Here's how the part is built. I have some questions about the finished solid (model axes, mm). A direction names the side the tool comes from. Coordinates: 2 decimals unless noted, no trailing zeros. Order: outer loops, then holes, each group sorted by start corner. A loop starts at its lowest first (then second) coordinate and runs counter-clockwise, first axis right, second up. Notation, with made-up numbers: (-39.75, 6) -> (-13.75, 6) arc R7 ccw to (-13.75, 10) -> close; hole circle Ø9 at (44.5, 80.5). An arc over 180 degrees is marked (long way). One line per item, written item: value. Start each with the question number.
```python
from build123d import *

# Parameters (mm, degrees)
F0_W     = 89.816496
F0_H     = 44.908248
F0_R     = 5.334
F1_DEPTH = 13.72113
F2_DEPTH = 25.4


with BuildPart() as f1:
    # F0 (on Front) → F1 (new body)
    with BuildSketch(Plane.XZ):
        with Locations((3.849279, -3.66598)):
            Rectangle(F0_W, F0_H)
        with Locations((-17.018, 0)):
            Circle(F0_R, mode=Mode.SUBTRACT)
        with Locations((17.018, 0)):
            Circle(F0_R, mode=Mode.SUBTRACT)
        with Locations((-17.018, 0)):
            Circle(F0_R)
        with Locations((17.018, 0)):
            Circle(F0_R)
    extrude(amount=F1_DEPTH)

    # F0 (on Front) → F2 (join)
    with BuildSketch(Plane.XZ):
        with Locations((17.018, 0)):
            Circle(F0_R)
        with Locations((-17.018, 0)):
            Circle(F0_R)
    extrude(amount=F2_DEPTH)


solid = f1.part
```
Q1. Imagine slicing it at A-A (z = 0). Write out the boundary of the cut face in (x, y), plus the area to 3 significant figures.
Q2. For faces 5 (the face through (11.69, -19.48, 0.23)), 6 (the face through (3, -7, 18.788)), which set-ups out of +Z, -Z, +X, -X, +Y, -Y let a thin tool reach every point of the face, with its end or its side?
Q3. If we mould it in two halves opening along X, with no side actions, what happens to faces 1 (the face through (-41.059, -7, -4)), 2 (the face through (-22.347, -19.479, 0.235)), 3 (the face through (48.758, -7, -4)), 4 (the face through (17, -25.4, 0))? For each: +X half, -X half, draft (parallel to the pull), parting line (faces both ways), or undercut.
Q4. I need wall thicknesses on line 1 (Y direction, x = 10.5, z = 6); line 2 (Z direction, x = -12.5, y = -18); line 3 (Z direction, x = 17.5, y = -21). Which ranges of each line are inside material? Lowest first, please.
Q5. Imagine slicing it at C-C (y = -22.25). Write out the boundary of the cut face in (x, z).
Q6. Imagine slicing it at D-D (z = -14.5). Write out the boundary of the cut face in (x, y).
Q7. For P1, Ø8, axis at y = -21.5, z = -2.5, coming from the -X side; P2, Ø5, axis at x = -0.5, z = -12.5, coming from the -Y side, each with a flat end and sliding along its axis, tell me the tip position at first contact or that it passes through.
Q8. Imagine slicing it at B-B (x = 18.5). Write out the boundary of the cut face in (y, z), plus the area to 3 significant figures.
Completed:
1. outline: (-41.06, -13.72) -> (-22.35, -13.72) -> (-22.35, -25.4) -> (-11.68, -25.4) -> (-11.68, -13.72) -> (11.68, -13.72) -> (11.68, -25.4) -> (22.35, -25.4) -> (22.35, -13.72) -> (48.76, -13.72) -> (48.76, 0) -> (-41.06, 0) -> close
1. area: 1,480 mm2
2. face 5: -Y
2. face 6: +Z, +X, -X, +Y, -Y
3. face 1: -X half
3. face 2: undercut
3. face 3: +X half
3. face 4: draft
4. line 1: y = -13.72 to 0
4. line 2: z = -2.84 to 2.84
4. line 3: z = -5.31 to 5.31
5. outline: circle Ø10.67 at (-17.02, 0); circle Ø10.67 at (17.02, 0)
6. outline: (-41.06, -13.72) -> (48.76, -13.72) -> (48.76, 0) -> (-41.06, 0) -> close
7. P1: stops at x = -22.35
7. P2: stops at y = -13.72
8. outline: (-25.4, -5.12) -> (-13.72, -5.12) -> (-13.72, -26.12) -> (0, -26.12) -> (0, 18.79) -> (-13.72, 18.79) -> (-13.72, 5.12) -> (-25.4, 5.12) -> close
8. area: 736 mm2
